Read the model definition and answer for the solid it produces. Units are mm, in the model's axes. Face numbers are marked on the shaded views. Round coordinates to 2 decimals unless told otherwise and drop trailing zeros. Write each loop counter-clockwise with the first axis right and the second up, starting at its lowest first coordinate (ties: lowest second). Pieces come first, ordered by that corner, then holes. Notation, with made-up numbers: (-2, 62) - (19, 62) arc R22 cw to (19, 73) - close; hole circle Ø1 at (36, -27.75). An arc over 180 degrees is marked (long way). Use one line per item in the form item = value. Start each with the question number.
1) For a pull along X with two mould halves and no side action, classify the marked faces 1, 2 and 3 as released by +X, released by -X, zero draft, split by the parting line, or undercut.
2) The part is cut by section B-B, the plane y = 0. Give the vertices of the cut face in (x, z).
3) The part is cut by section C-C, the plane y = 19. Give the vertices of the cut face in (x, z).
4) The part is cut by section D-D, the plane x = 23. Give the vertices of the cut face in (y, z), plus the area to 3 significant figures.
5) Consider line 1 along X through (y, z) = (-5, 2); line 2 along X through (y, z) = (0, 2); line 3 along Y through (x, z) = (-9, 1.75). Determine where each line is inside the solid, lowest interval first. Write a range as from..to.
6) Each of these flat-tipped pins is pushed along its axis until it touches: pin 1 (3 mm diameter, centred on x = 8.5, z = 0.5, fed in from +Y); pin 2 (0.6 mm diameter, centred on y = -14, z = -1, fed in from -X); pin 3 (1.3 mm diameter, centred on x = 12, z = -1, fed in from +Y). Where does it stop, or does it pass through?
from build123d import *

# Parameters (mm, degrees)
F0_R     = 11.15
F1_DEPTH = 3.5
F3_DEPTH = 6


with BuildPart() as f1:
    # F0 (on Top) → F1 (new body, symmetric)
    with BuildSketch(Plane.XY):
        Polygon((-29.073366, -20.207259), (29.073366, -20.207259), (32.036683, -15.074644), (2.963317, 35.281903), (-2.963317, 35.281903), (-32.036683, -15.074644), align=None)
        Circle(F0_R, mode=Mode.SUBTRACT)
    extrude(amount=F1_DEPTH, both=True)

    # F2 (on face) → F3 (cut)
    with BuildSketch(Plane.XY.offset(3.5)):
        Polygon((14.704705, 2.253575), (10.919886, 2.253575), (10.919886, 1.753575), (15.282055, 1.753575), (15.282055, 2.253575), align=None)
        Polygon((0, 27.722871), (14.704705, 2.253575), (15.282055, 2.253575), (0.433013, 27.972871), align=None)
        Polygon((-9.304005, 11.607861), (-9.592681, 12.107861), (-24.441723, -13.611435), (-24.00871, -13.861435), align=None)
        Polygon((-9.159668, 12.357861), (-9.592681, 12.107861), (-9.304005, 11.607861), (-7.411596, 8.330111), (-6.978583, 8.580111), align=None)
        Polygon((-5.4007, -13.861435), (-5.689375, -14.361435), (24.00871, -14.361435), (24.00871, -13.861435), align=None)
        Polygon((-6.122387, -14.111435), (-5.689375, -14.361435), (-5.4007, -13.861435), (-3.50829, -10.583686), (-3.941303, -10.333686), align=None)
    extrude(amount=-F3_DEPTH, mode=Mode.SUBTRACT)


solid = f1.part
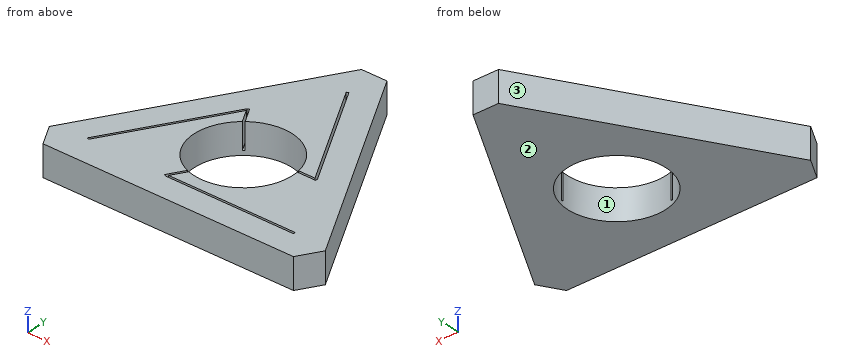
Geometry results:
q1.face_1 = undercut
q1.face_2 = zero draft
q1.face_3 = released by -X
q2.outline = (-23.33, -3.5) - (-11.15, -3.5) - (-11.15, 3.5) - (-16.01, 3.5) - (-16.01, -2.5) - (-16.58, -2.5) - (-16.58, 3.5) - (-23.33, 3.5) - close; (11.15, -3.5) - (23.33, -3.5) - (23.33, 3.5) - (11.15, 3.5) - close
q3.outline = (-12.36, -3.5) - (12.36, -3.5) - (12.36, 3.5) - (5.61, 3.5) - (5.61, -2.5) - (5.04, -2.5) - (5.04, 3.5) - (-12.36, 3.5) - close
q4.outline = (-20.21, -3.5) - (0.58, -3.5) - (0.58, 3.5) - (-13.86, 3.5) - (-13.86, -2.5) - (-14.36, -2.5) - (-14.36, 3.5) - (-20.21, 3.5) - close
q4.area = 142 mm2
q5.line_1 = -26.22..-19.47, -18.89..-9.97, 9.97..26.22
q5.line_2 = -23.33..-16.58, -16.01..-11.15, 11.15..23.33
q5.line_3 = -20.21..-6.58, 6.58..11.08, 12.08..24.83
q6.pin_1 = 28.29
q6.pin_2 = -31.59
q6.pin_3 = 20.76
